For this review, use the dimensioned drawing (mm, ordinates from the lowest corner) and the shaded views. A direction names the side the tool comes from. Give positions to 0.01 mm unless a question says otherwise; leave off trailing zeros. Loops run counter-clockwise (first coordinate to the right, second up) from the corner with the lowest first, then second, coordinate; pieces in that order, holes last. Notation, with made-up numbers: (70, 64) - (97, 64) arc R13 ccw to (97, 69) - close; hole circle Ø5 at (11.25, 72). An arc over 180 degrees is marked (long way). Write each question's results on one line, items separated by ' | '.
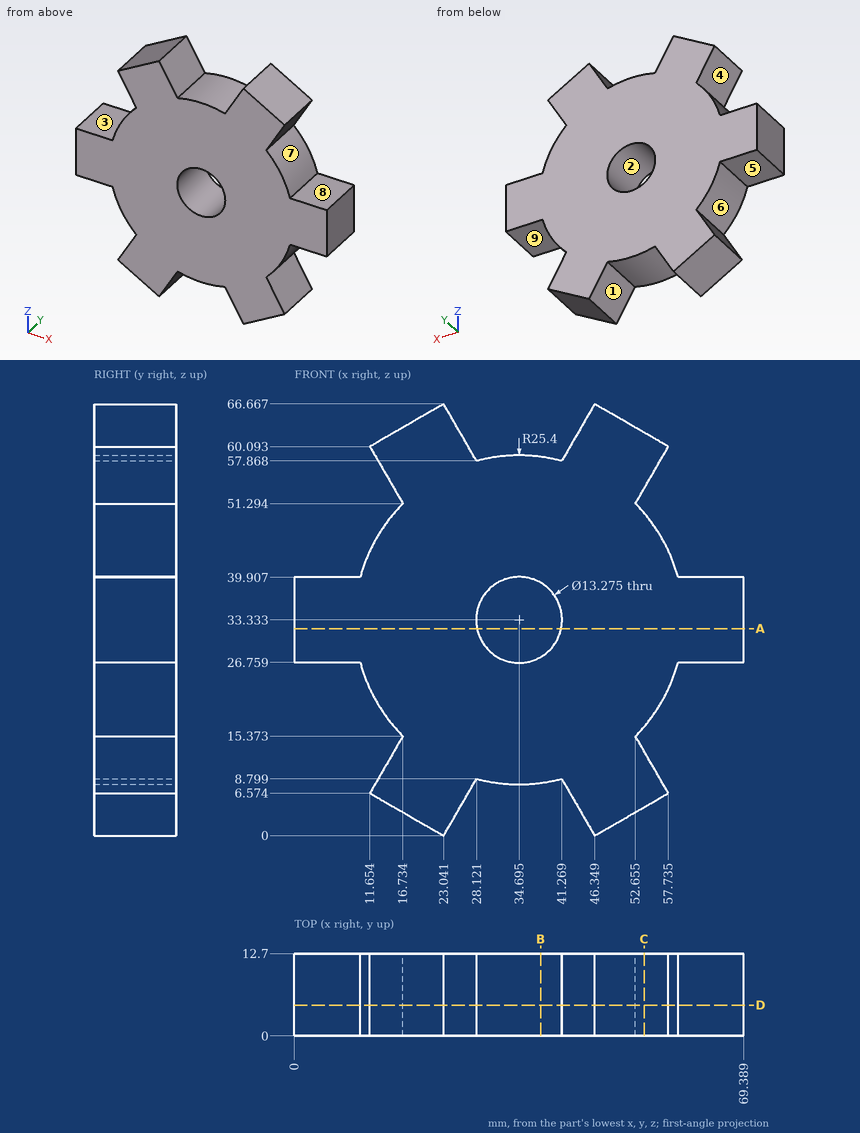
Item 1: Wall thickness on probe 1 along X at (y, z) = (5.75, 33) (1 decimal); probe 2 along Z at (x, y) = (4.5, 6.5); probe 3 along Z at (x, y) = (55, 2.25) (1 decimal): over which ranges is each line inside the solid? List them lowest first.
Output values:
probe 1: x = 0 to 28.1, 41.3 to 69.4 | probe 2: z = 26.76 to 39.91 | probe 3: z = 5 to 11.3, 18.1 to 48.6, 55.4 to 61.7
Item 2: We need section B-B on x = 38. Give the boundary of the cut face in (y, z).
Output values:
outline: (0, 8.15) - (12.7, 8.15) - (12.7, 27.58) - (0, 27.58) - close; (0, 39.09) - (12.7, 39.09) - (12.7, 58.52) - (0, 58.52) - close
Item 3: We need section C-C on x = 54. Give the boundary of the cut face in (y, z).
Output values:
outline: (0, 4.42) - (12.7, 4.42) - (12.7, 13.04) - (0, 13.04) - close; (0, 16.83) - (12.7, 16.83) - (12.7, 49.84) - (0, 49.84) - close; (0, 53.62) - (12.7, 53.62) - (12.7, 62.25) - (0, 62.25) - close
Item 4: Draft analysis for pull direction X (two halves, no side actions). For the marked faces 1, 2, 3 and 4, state which applies: +X half, -X half, draft (parallel to the pull), parting line (faces both ways), or undercut.
Output values:
face 1: undercut | face 2: undercut | face 3: draft | face 4: -X half
Item 5: Tool access review of the marked faces 5, 6, 7, 8 and 9: name each direction out of +Z, -Z, +X, -X, +Y, -Y from which nothing blocks a thin tool from reaching the whole face with its end or side.
Output values:
face 5: -Z, -X, +Y, -Y | face 6: -X, +Y, -Y | face 7: +X, +Y, -Y | face 8: +Z, +X, +Y, -Y | face 9: -Z, +X, +Y, -Y
Item 6: We need section D-D on y = 4.75. Give the boundary of the cut face in (x, z) (1 decimal), then the cut area to 3 significant figures.
Output values:
outline: (0, 26.8) - (10.2, 26.8) arc R25.4 ccw to (16.7, 15.4) - (11.7, 6.6) - (23, 0) - (28.1, 8.8) arc R25.4 ccw to (41.3, 8.8) - (46.3, 0) - (57.7, 6.6) - (52.7, 15.4) arc R25.4 ccw to (59.2, 26.8) - (69.4, 26.8) - (69.4, 39.9) - (59.2, 39.9) arc R25.4 ccw to (52.7, 51.3) - (57.7, 60.1) - (46.3, 66.7) - (41.3, 57.9) arc R25.4 ccw to (28.1, 57.9) - (23, 66.7) - (11.7, 60.1) - (16.7, 51.3) arc R25.4 ccw to (10.2, 39.9) - (0, 39.9) - close; hole circle Ø13.3 at (34.7, 33.3) | area: 2,640 mm²
Item 7: We need section A-A on z = 32. Give the boundary of the cut face in (x, y), then the cut area to 3 significant figures.
Output values:
outline: (0, 0) - (28.19, 0) - (28.19, 12.7) - (0, 12.7) - close; (41.2, 0) - (69.39, 0) - (69.39, 12.7) - (41.2, 12.7) - close | area: 716 mm²
Item 8: Clearance check with flat-ended pins moving along their axes: P1, Ø5, axis at x = 64.5, y = 4, coming from the -Z side; P2, Ø1, axis at y = 8, z = 57.5, coming from the +X side; P3, Ø5, axis at x = 66.5, y = 9, coming from the +Z side. State where each tip first meets the part, or that it passes through.
Output values:
P1: stops at z = 26.76 | P2: stops at x = 56.53 | P3: stops at z = 39.91
